Geometry check sheet. Reference: the model listing, model coordinates, mm. Face numbers are marked on the shaded views. A direction names the side the tool comes from. Coordinates: 2 decimals unless noted, no trailing zeros. Order: outer loops, then holes, each group sorted by start corner. A loop starts at its lowest first (then second) coordinate and runs counter-clockwise, first axis right, second up. Notation, with made-up numbers: (-25.5, -1) - (-10.5, -1) arc R27 ccw to (-10.5, 29) - close; hole circle Ø6 at (78.25, 69.5). An arc over 180 degrees is marked (long way). Use CSV: the item, a comma, the result in double quotes. Start each with the question number.
1) Tool access check on the marked faces 1 and 2. Record the directions out of +Z, -Z, +X, -X, +Y, -Y that give a thin tool (end or side, any length) a straight path to the whole face; none if there is none.
2) Sectioned sample at A-A, the plane y = 22.5. Record the cut outline in (x, z).
3) Sectioned sample at D-D, the plane y = -34. Record the cut outline in (x, z).
4) Sectioned sample at B-B, the plane z = -3. Count the separate pieces of the cut face and the enclosed holes in it, and give its area (3 significant figures).
5) Thickness scan on probe 1 along Y at (x, z) = (0, -9.4); probe 2 along Y at (x, z) = (0, -1.3); probe 3 along X at (y, z) = (11.25, -6.5). Record the ranges inside material, lowest first. Write a range as [from, to].
6) Depth check by flat-ended pin: P1, Ø22, axis at x = 1, y = 0, coming from the +Z side; P2, Ø6, axis at x = -14.5, z = -9, coming from the +Y side; P3, Ø9, axis at x = -1, y = 7.5, coming from the -Z side; P4, Ø8, axis at x = -9, y = -36, coming from the +Z side. Enter the tip coordinate at first touch or a pass-through.
7) Sectioned sample at C-C, the plane y = -54.5. Record the cut outline in (x, z), and give its area (3 significant figures).
8) Draft check along Y on the marked faces 3, 4, 5 and 6. Enter one of: released by +Y, released by -Y, zero draft, split by the parting line, or undercut.
from build123d import *

# Parameters (mm, degrees)
SKETCH_2_R                   = 25
EXTRUDE_2_DEPTH              = 4
SKETCH_22_R                  = 10
CUT_EXTRUDE_1_DEPTH          = 2
FILLET_4_R                   = 0.2
SKETCH_54_R                  = 25
EXTRUDE_6_DEPTH              = 11
SKETCH_55_R                  = 18.5
CUT_EXTRUDE_2_DEPTH          = 10
HOLE_WIZARD_M4_1_D           = 4.5
HOLE_WIZARD_M4_1_CBORE_D     = 8
HOLE_WIZARD_M4_1_CBORE_DEPTH = 1
PATTERN_CIRCULAR_1_COUNT     = 3
SKETCH_59_R                  = 18.5
SKETCH_59_R_2                = 17.5
EXTRUDE_7_DEPTH              = 1
EXTRUDE_START                = -9
EXTRUDE_8_DEPTH              = 9
FILLET_6_R                   = 0.3
SKETCH_68_R                  = 9.5
CUT_EXTRUDE_7_DEPTH          = 7
SKETCH_69_R                  = 8.5
CUT_EXTRUDE_8_DEPTH          = 2
CUT_EXTRUDE_START            = -75
SKETCH_80_W                  = 72.028937147
SKETCH_80_H                  = 9.617570508
CUT_EXTRUDE_9_DEPTH          = 100
EXTRUDE_START_2              = -2
SKETCH_82_R                  = 9.5
SKETCH_82_R_2                = 8.5
EXTRUDE_9_DEPTH              = 2
PATTERN_CIRCULAR_2_COUNT     = 6


with BuildPart() as part:
    # Sketch 2 → Extrude 2 (new body)
    with BuildSketch(Plane(origin=(0, 6, 0), x_dir=(1, 0, 0), z_dir=(0, 0, -1))):
        with Locations((0, 6)):
            Circle(SKETCH_2_R)
    extrude(amount=EXTRUDE_2_DEPTH)

    # Sketch 22 → Cut-Extrude 1 (cut)
    with BuildSketch(Plane.XY):
        Circle(SKETCH_22_R)
    extrude(amount=-CUT_EXTRUDE_1_DEPTH, mode=Mode.SUBTRACT)

    # Fillet 4
    fillet_4_edges = [part.edges().sort_by_distance(p)[0] for p in [
        (-10, 0, 0),
    ]]
    fillet(fillet_4_edges, radius=FILLET_4_R)

    # Sketch 54 → Extrude 6 (add)
    with BuildSketch(Plane(origin=(0, 0, -4), x_dir=(-1, 0, 0), z_dir=(0, 0, -1))):
        Circle(SKETCH_54_R)
    extrude(amount=EXTRUDE_6_DEPTH)

    # Sketch 55 → Cut-Extrude 2 (cut)
    with BuildSketch(Plane(origin=(0, 0, -15), x_dir=(-1, 0, 0), z_dir=(0, 0, -1))):
        Circle(SKETCH_55_R)
    extrude(amount=-CUT_EXTRUDE_2_DEPTH, mode=Mode.SUBTRACT)

    # Hole Wizard M4 _ _ _ _ _ _1 (through all)
    with Locations(Plane(origin=(0, 0, -5), x_dir=(-1, 0, 0), z_dir=(0, 0, -1))):
        with Locations((0, 7)):
            hole_wizard_m4_1 = CounterBoreHole(HOLE_WIZARD_M4_1_D / 2, HOLE_WIZARD_M4_1_CBORE_D / 2, HOLE_WIZARD_M4_1_CBORE_DEPTH)

    # Pattern Circular 1: Hole Wizard M4 _ _ _ _ _ _1 ×3 about axis
    pattern_circular_1_axis = Axis((0, 0, 0), (0, 0, 1))
    for i in range(1, PATTERN_CIRCULAR_1_COUNT):
        add(hole_wizard_m4_1.rotate(pattern_circular_1_axis, i * 360 / PATTERN_CIRCULAR_1_COUNT), mode=Mode.SUBTRACT)

    # Sketch 59 → Extrude 7 (add)
    with BuildSketch(Plane(origin=(0, 0, -5), x_dir=(-1, 0, 0), z_dir=(0, 0, -1))):
        Circle(SKETCH_59_R)
        Circle(SKETCH_59_R_2, mode=Mode.SUBTRACT)
    extrude(amount=EXTRUDE_7_DEPTH)

    # Sketch 60 → Extrude 8 (add)
    with BuildSketch(Plane(origin=(0, 0, -15), x_dir=(-1, 0, 0), z_dir=(0, 0, -1)).offset(EXTRUDE_START)):
        with BuildLine():
            Line((-24.65033243, -4.166666667), (-14.790199458, -62.5))
            ThreePointArc((-14.790199458, -62.5), (0, -75), (14.790199458, -62.5))
            Line((14.790199458, -62.5), (24.65033243, -4.166666667))
            ThreePointArc((24.65033243, -4.166666667), (0, -25), (-24.65033243, -4.166666667))
        make_face()
    extrude(amount=EXTRUDE_8_DEPTH)

    # Fillet 6
    fillet_6_edges = [part.edges().sort_by_distance(p)[0] for p in [
        (18.5, 0, -6),
    ]]
    fillet(fillet_6_edges, radius=FILLET_6_R)

    # Sketch 68 → Cut-Extrude 7 (cut)
    with BuildSketch(Plane.XY.offset(-6)):
        with Locations((0, -60)):
            Circle(SKETCH_68_R)
    extrude(amount=-CUT_EXTRUDE_7_DEPTH, mode=Mode.SUBTRACT)

    # Sketch 69 → Cut-Extrude 8 (cut)
    with BuildSketch(Plane.XY.offset(-13)):
        with Locations((0, -60)):
            Circle(SKETCH_69_R)
    extrude(amount=-CUT_EXTRUDE_8_DEPTH, mode=Mode.SUBTRACT)

    # Sketch 80 → Cut-Extrude 9 (cut)
    with BuildSketch(Plane(origin=(0, 0, 0), x_dir=(1, 0, 0), z_dir=(0, 1, 0)).offset(CUT_EXTRUDE_START)):
        with Locations((0.446829634, 14.808785254)):
            Rectangle(SKETCH_80_W, SKETCH_80_H)
    extrude(amount=CUT_EXTRUDE_9_DEPTH, mode=Mode.SUBTRACT)

    # Sketch 82 → Extrude 9 (add)
    with BuildSketch(Plane.XY.offset(-6).offset(EXTRUDE_START_2)):
        with Locations((0, -60)):
            Circle(SKETCH_82_R)
        with Locations((0, -60)):
            Circle(SKETCH_82_R_2, mode=Mode.SUBTRACT)
    extrude(amount=EXTRUDE_9_DEPTH)

    # Sketch 87 → Hole Wizard M3 _ _ _ _1 (revolve, cut)
    with BuildSketch(Plane(origin=(0, 22.5, -10), x_dir=(0, 1, 0), z_dir=(1, 0, 0))):
        Polygon((0, 0), (0, 222.751075774), (1.25, 222), (1.25, 0), align=None)
    hole_wizard_m3_1 = revolve(axis=Axis((0, 22.5, -16.35), (0, 0, 1)), mode=Mode.SUBTRACT)

    # Pattern Circular 2: Hole Wizard M3 _ _ _ _1 ×6 about axis
    pattern_circular_2_axis = Axis((0, 0, 0), (0, 0, 1))
    for i in range(1, PATTERN_CIRCULAR_2_COUNT):
        add(hole_wizard_m3_1.rotate(pattern_circular_2_axis, i * 360 / PATTERN_CIRCULAR_2_COUNT), mode=Mode.SUBTRACT)


solid = part.part
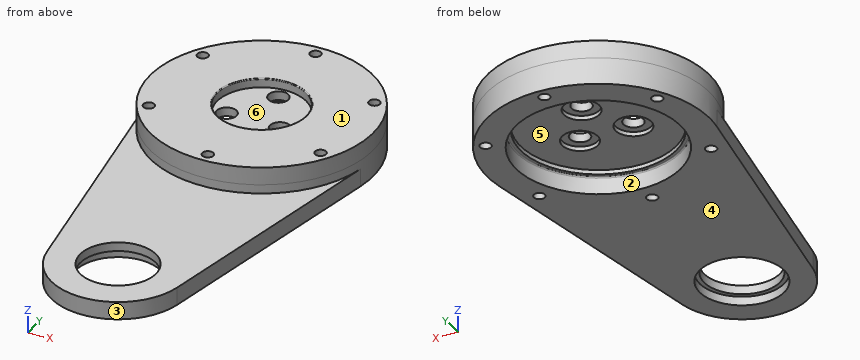
Evaluation:
1,face 1,"+Z, +X, -X, +Y, -Y"
1,face 2,"-Z"
2,outline,"(-10.9, -10) - (-1.25, -10) - (-1.25, 0) - (-10.9, 0) - close; (1.25, -10) - (10.9, -10) - (10.9, 0) - (1.25, 0) - close"
3,outline,"(-19.61, -10) - (19.61, -10) - (19.61, -6) - (-19.61, -6) - close"
4,separate pieces,"1"
4,enclosed holes,"9"
4,area,"1,890 mm²"
5,probe 1,"[-75, -69.5], [-50.5, -23.75], [-21.25, -18.5], [18.5, 21.25], [23.75, 25]"
5,probe 2,"[-25, -23.75], [-21.25, -10], [10, 21.25], [23.75, 25]"
5,probe 3,"[-22.33, -20.74], [-18.24, -14.69], [14.69, 18.24], [20.74, 22.33]"
6,P1,"z = 0"
6,P2,"y = 22.2"
6,P3,"z = -5"
6,P4,"z = -6"
7,outline,"(-16.14, -10) - (-7.75, -10) - (-7.75, -8) - (-6.48, -8) - (-6.48, -6) - (-16.14, -6) - close; (6.48, -8) - (7.75, -8) - (7.75, -10) - (16.14, -10) - (16.14, -6) - (6.48, -6) - close"
7,area,"72.2 mm²"
8,face 3,"released by -Y"
8,face 4,"zero draft"
8,face 5,"undercut"
8,face 6,"undercut"
